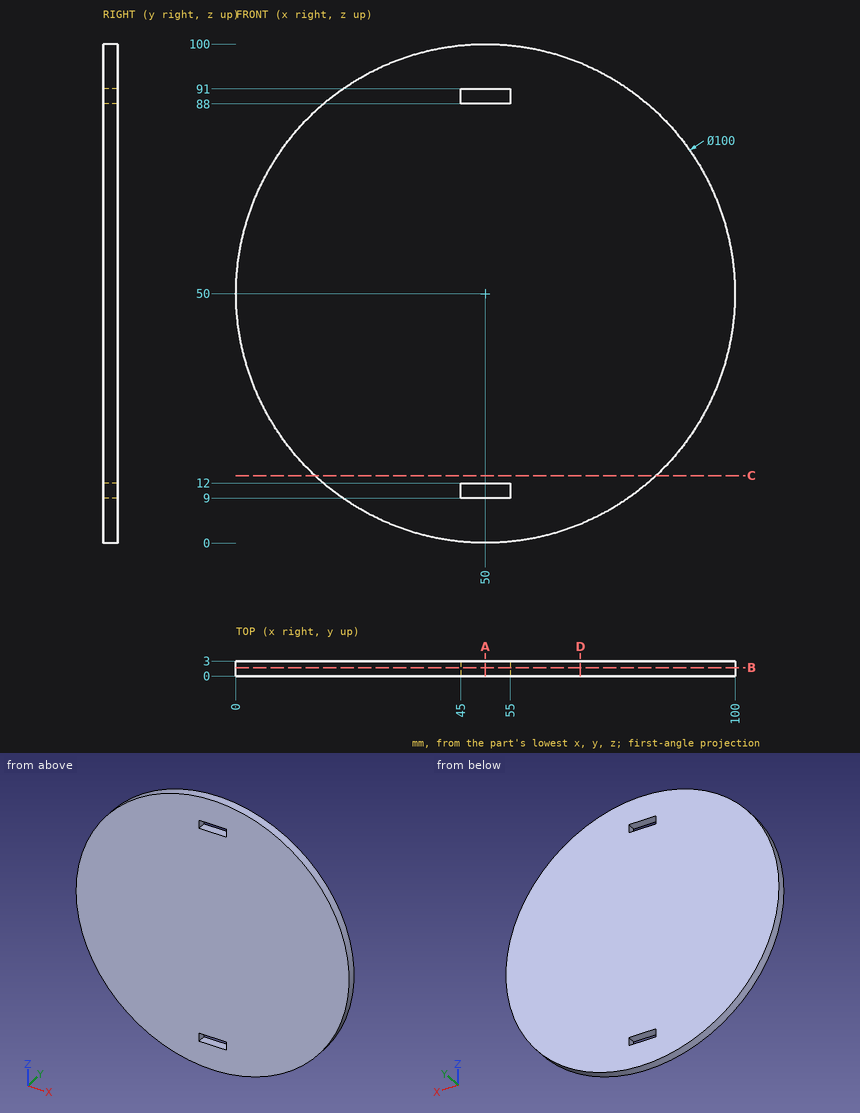
Answer from the drawing. Dimensions are ordinates in mm from the lowest x, y and z of the part. Round coordinates to 2 decimals unless told otherwise and drop trailing zeros. Loops run counter-clockwise (first coordinate to the right, second up) from the corner with the lowest first, then second, coordinate; pieces in that order, holes last. Notation, with made-up numbers: M 88,17 L 99,17 A29 ccw 99,47 Z; hole C 80,44 d9. An arc over 180 degrees is marked long. One line per question, with ' | ' between items. Start each with the question number.
(1) A cutting plane is placed at B-B on y = 1.7. Write down the section's boundary in (x, z).
(2) Flat-ended cylindrical pins translate along their axes: pin 1 Ø0.9 at (x, y) = (51, 1) entering from -Z; pin 2 Ø1.5 at (x, y) = (52, 1) entering from +Z; pin 3 Ø0.9 at (y, z) = (1.5, 89) entering from -X. Find the tip coordinate at first contact, or state that the pin passes through.
(3) A cutting plane is placed at A-A on x = 50. Write down the section's boundary in (y, z), plus the area to 3 significant figures.
(4) Find the intervals of material crossed by line 1 (Z direction, x = 52.5, y = 0.85); line 2 (Z direction, x = 52, y = 2.35); line 3 (X direction, y = 0.55, z = 11), in increasing order.
(5) A cutting plane is placed at C-C on z = 13.5. Write down the section's boundary in (x, y), plus the area to 3 significant figures.
(6) A cutting plane is placed at D-D on x = 69. Write down the section's boundary in (y, z), plus the area to 3 significant figures.
Geometry check:
1) outline: C 50,50 d100; hole M 45,9 L 55,9 L 55,12 L 45,12 Z; hole M 45,88 L 55,88 L 55,91 L 45,91 Z
2) pin 1: stops at z = 0 | pin 2: stops at z = 99.98 | pin 3: stops at x = 18.16
3) outline: M 0,0 L 3,0 L 3,9 L 0,9 Z; M 0,12 L 3,12 L 3,88 L 0,88 Z; M 0,91 L 3,91 L 3,100 L 0,100 Z | area: 282 mm²
4) line 1: z = 0.06 to 9, 12 to 88, 91 to 99.94 | line 2: z = 0.04 to 9, 12 to 88, 91 to 99.96 | line 3: x = 18.71 to 45, 55 to 81.29
5) outline: M 15.83,0 L 84.17,0 L 84.17,3 L 15.83,3 Z | area: 205 mm²
6) outline: M 0,3.75 L 3,3.75 L 3,96.25 L 0,96.25 Z | area: 277 mm²
